from build123d import *

# Parameters (mm, degrees)
F0_R     = 1.5
F1_DEPTH = 48
F2_R     = 11
F2_R_2   = 4
F3_DEPTH = 2
F4_R     = 2.5
F5_DEPTH = 24


with BuildPart() as f1:
    # F0 (on Top) → F1 (new body)
    with BuildSketch(Plane.XY):
        Polygon((-21, 17), (-21, 0), (-21, -17), (-17, -21), (0, -21), (17, -21), (21, -17), (21, 0), (21, 17), (17, 21), (0, 21), (-17, 21), align=None)
        with Locations((-15.5, -15.5)):
            Circle(F0_R, mode=Mode.SUBTRACT)
        with Locations((15.5, -15.5)):
            Circle(F0_R, mode=Mode.SUBTRACT)
        with Locations((-15.5, 15.5)):
            Circle(F0_R, mode=Mode.SUBTRACT)
        with Locations((15.5, 15.5)):
            Circle(F0_R, mode=Mode.SUBTRACT)
    extrude(amount=-F1_DEPTH)

    # F2 (on face) → F3 (join)
    with BuildSketch(Plane.XY):
        Circle(F2_R)
        Circle(F2_R_2, mode=Mode.SUBTRACT)
    extrude(amount=F3_DEPTH)

    # F4 (on face) → F5 (join)
    with BuildSketch(Plane.XY):
        Circle(F4_R)
    extrude(amount=F5_DEPTH)


solid = f1.part
Work out the finished part from the listing and answer in its coordinate system (mm). A direction names the side the tool comes from. Give positions to 0.01 mm unless a question says otherwise; leave off trailing zeros. Loops run counter-clockwise (first coordinate to the right, second up) from the corner with the lowest first, then second, coordinate; pieces in that order, holes last. Notation, with made-up numbers: (12.25, -32) -> (67.25, -32) arc R19 ccw to (67.25, 5) -> close; hole circle Ø4 at (14, 71). An arc over 180 degrees is marked (long way). Use a Markdown table: item, result. Add a question column.
1. For faces 4 (the flat face through (19, -19, -24)), 5 (the flat face through (-10, -9, 0)), determine the directions among +Z, -Z, +X, -X, +Y, -Y from which every point of the face is accessible in a straight line to the end or side of a thin tool.
2. Determine the mould class of faces 1 (the flat face through (-19, 19, -24)), 2 (the cylindrical face through (-2.38, -10.74, 0.99)), 3 (the flat face through (-2, -2, 0)) for opening direction Y: released by +Y, released by -Y, zero draft, split by the parting line, or undercut.
3. Find the intervals of material crossed by probe 1 along Y at (x, z) = (15.5, -31.5); probe 2 along X at (y, z) = (-15, -16); probe 3 along Z at (x, y) = (-12.5, -18), in increasing order.
4. Section D-D on x = 0 is taken. Determine the outline of the cut face in (y, z), and give its area (3 significant figures).
5. Section B-B on z = 1 is taken. Determine the outline of the cut face in (x, y).
6. Flat-ended cylindrical pins translate along their axes: pin 1 Ø24 at (x, y) = (2, -4.5) entering from +Z; pin 2 Ø1 at (x, y) = (16.5, 15) entering from +Z; pin 3 Ø2 at (x, y) = (-7.5, 5.5) entering from +Z. Find the tip coordinate at first contact, or state that the pin passes through.
7. Section A-A on x = 15.5 is taken. Determine the outline of the cut face in (y, z), and give its area (3 significant figures).
Results below:
| question | item | result |
|---|---|---|
| 1 | face 4 | +Z, -Z, +X, -Y |
| 1 | face 5 | +Z |
| 2 | face 1 | released by +Y |
| 2 | face 2 | split by the parting line |
| 2 | face 3 | undercut |
| 3 | probe 1 | y = -21 to -17, -14 to 14, 17 to 21 |
| 3 | probe 2 | x = -21 to -16.91, -14.09 to 14.09, 16.91 to 21 |
| 3 | probe 3 | z = -48 to 0 |
| 4 | outline | (-21, -48) -> (21, -48) -> (21, 0) -> (11, 0) -> (11, 2) -> (4, 2) -> (4, 0) -> (2.5, 0) -> (2.5, 24) -> (-2.5, 24) -> (-2.5, 0) -> (-4, 0) -> (-4, 2) -> (-11, 2) -> (-11, 0) -> (-21, 0) -> close |
| 4 | area | 2,160 mm^2 |
| 5 | outline | circle Ø22 at (0, 0); circle Ø5 at (0, 0); hole circle Ø8 at (0, 0) |
| 6 | pin 1 | stops at z = 24 |
| 6 | pin 2 | stops at z = 0 |
| 6 | pin 3 | stops at z = 2 |
| 7 | outline | (-21, -48) -> (-17, -48) -> (-17, 0) -> (-21, 0) -> close; (-14, -48) -> (14, -48) -> (14, 0) -> (-14, 0) -> close; (17, -48) -> (21, -48) -> (21, 0) -> (17, 0) -> close |
| 7 | area | 1,730 mm^2 |
